Geometry check sheet. Reference: the model listing, model coordinates, mm. Face numbers are marked on the shaded views. A direction names the side the tool comes from. Coordinates: 2 decimals unless noted, no trailing zeros. Order: outer loops, then holes, each group sorted by start corner. A loop starts at its lowest first (then second) coordinate and runs counter-clockwise, first axis right, second up. Notation, with made-up numbers: (38.25, 68) - (96.25, 68) arc R13 cw to (96.25, 86) - close; hole circle Ø3 at (14.5, 17.25). An arc over 180 degrees is marked (long way). Use CSV: the item, a comma, the result in double quotes. Start each with the question number.
1) Sectioned sample at C-C, the plane z = 4. Record the cut outline in (x, y).
2) Thickness scan on probe 1 along X at (y, z) = (0.8, 19.5); probe 2 along Z at (x, y) = (-20, 1.9); probe 3 along Y at (x, z) = (17.5, -19.5). Record the ranges inside material, lowest first. Write a range as [from, to].
3) Sectioned sample at A-A, the plane y = 3.05. Record the cut outline in (x, z), and give its area (3 significant figures).
4) Depth check by flat-ended pin: P1, Ø0.6, axis at y = 2.5, z = -0.5, coming from the +X side; P2, Ø2.5, axis at x = 19.5, z = -19.5, coming from the +Y side. Enter the tip coordinate at first touch or a pass-through.
5) Tool access check on the marked faces 1 and 2. Record the directions out of +Z, -Z, +X, -X, +Y, -Y that give a thin tool (end or side, any length) a straight path to the whole face; none if there is none.
6) Sectioned sample at B-B, the plane y = 0.7. Record the cut outline in (x, z).
7) Sectioned sample at D-D, the plane x = 5.5. Record the cut outline in (y, z), and give its area (3 significant figures).
from build123d import *

# Parameters (mm, degrees)
SKETCH2_R           = 1.5
BOSS_EXTRUDE1_DEPTH = 2
BOSS_EXTRUDE2_DEPTH = 2
CUT_EXTRUDE1_DEPTH  = 2


with BuildPart() as part:
    # Sketch2 → Boss-Extrude1 (new body)
    with BuildSketch(Plane(origin=(0, 0, 0), x_dir=(1, 0, 0), z_dir=(0, 1, 0))):
        with BuildLine():
            Line((-19.5, 22.5), (19.5, 22.5))
            ThreePointArc((19.5, 22.5), (21.621320344, 21.621320344), (22.5, 19.5))
            Line((22.5, 19.5), (22.5, -19.5))
            ThreePointArc((22.5, -19.5), (21.621320344, -21.621320344), (19.5, -22.5))
            Line((19.5, -22.5), (-19.5, -22.5))
            ThreePointArc((-19.5, -22.5), (-21.621320344, -21.621320344), (-22.5, -19.5))
            Line((-22.5, -19.5), (-22.5, 19.5))
            ThreePointArc((-22.5, 19.5), (-21.621320344, 21.621320344), (-19.5, 22.5))
        make_face()
        with Locations(Location((19.5, -19.5, 0), (0, 0, 270))):
            Circle(SKETCH2_R, mode=Mode.SUBTRACT)
        with Locations(Location((19.5, 19.5, 0), (0, 0, 270))):
            Circle(SKETCH2_R, mode=Mode.SUBTRACT)
        with Locations(Location((-19.5, 19.5, 0), (0, 0, 270))):
            Circle(SKETCH2_R, mode=Mode.SUBTRACT)
        with Locations(Location((-19.5, -19.5, 0), (0, 0, 270))):
            Circle(SKETCH2_R, mode=Mode.SUBTRACT)
    extrude(amount=BOSS_EXTRUDE1_DEPTH)

    # Sketch3 → Boss-Extrude2 (add)
    with BuildSketch(Plane(origin=(0, 2, 0), x_dir=(1, 0, 0), z_dir=(0, 1, 0))):
        with BuildLine():
            Line((-11.653247837, 14.653247837), (11.653247837, 14.653247837))
            ThreePointArc((11.653247837, 14.653247837), (13.774568181, 13.774568181), (14.653247837, 11.653247837))
            Line((14.653247837, 11.653247837), (14.653247837, -11.653247837))
            ThreePointArc((14.653247837, -11.653247837), (13.774568181, -13.774568181), (11.653247837, -14.653247837))
            Line((11.653247837, -14.653247837), (-11.653247837, -14.653247837))
            ThreePointArc((-11.653247837, -14.653247837), (-13.774568181, -13.774568181), (-14.653247837, -11.653247837))
            Line((-14.653247837, -11.653247837), (-14.653247837, 11.653247837))
            ThreePointArc((-14.653247837, 11.653247837), (-13.774568181, 13.774568181), (-11.653247837, 14.653247837))
        make_face()
    extrude(amount=BOSS_EXTRUDE2_DEPTH)

    # Sketch4 → Cut-Extrude1 (cut)
    with BuildSketch(Plane(origin=(0, 4, 0), x_dir=(1, 0, 0), z_dir=(0, 1, 0))):
        with BuildLine():
            Line((11.675246151, -1.309846963), (1.675246151, -2.488684458))
            ThreePointArc((1.675246151, -2.488684458), (0, -3), (-1.675246151, -2.488684458))
            Line((-1.675246151, -2.488684458), (-11.675246151, -1.309846963))
            ThreePointArc((-11.675246151, -1.309846963), (-12.444287238, 0), (-11.675246151, 1.309846963))
            Line((-11.675246151, 1.309846963), (-1.675246151, 2.488684458))
            ThreePointArc((-1.675246151, 2.488684458), (0, 3), (1.675246151, 2.488684458))
            Line((1.675246151, 2.488684458), (11.675246151, 1.309846963))
            ThreePointArc((11.675246151, 1.309846963), (12.444287238, 0), (11.675246151, -1.309846963))
        make_face()
    extrude(amount=-CUT_EXTRUDE1_DEPTH, mode=Mode.SUBTRACT)


solid = part.part
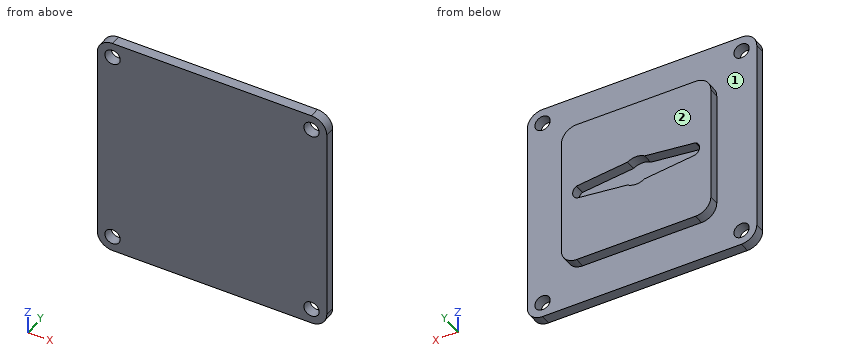
Evaluation:
1,outline,"(-22.5, 0) - (22.5, 0) - (22.5, 2) - (14.65, 2) - (14.65, 4) - (-14.65, 4) - (-14.65, 2) - (-22.5, 2) - close"
2,probe 1,"[-22.5, -21], [-18, 18], [21, 22.5]"
2,probe 2,"[-22.46, -20.91], [-18.09, 18.09], [20.91, 22.46]"
2,probe 3,"[0, 2]"
3,outline,"(-14.65, -11.65) arc R3 ccw to (-11.65, -14.65) - (11.65, -14.65) arc R3 ccw to (14.65, -11.65) - (14.65, 11.65) arc R3 ccw to (11.65, 14.65) - (-11.65, 14.65) arc R3 ccw to (-14.65, 11.65) - close; hole (-11.68, -1.31) - (-1.68, -2.49) arc R3 ccw to (1.68, -2.49) - (11.68, -1.31) arc R1.5 ccw to (11.68, 1.31) - (1.68, 2.49) arc R3 ccw to (-1.68, 2.49) - (-11.68, 1.31) arc R1.5 ccw to start"
3,area,"753 mm²"
4,P1,"x = 14.65"
4,P2,"through"
5,face 1,"+Y"
5,face 2,"+Z, -Z, +X, -X, +Y"
6,outline,"(-22.5, -19.5) arc R3 ccw to (-19.5, -22.5) - (19.5, -22.5) arc R3 ccw to (22.5, -19.5) - (22.5, 19.5) arc R3 ccw to (19.5, 22.5) - (-19.5, 22.5) arc R3 ccw to (-22.5, 19.5) - close; hole circle Ø3 at (-19.5, -19.5); hole circle Ø3 at (-19.5, 19.5); hole circle Ø3 at (19.5, -19.5); hole circle Ø3 at (19.5, 19.5)"
7,outline,"(0, -22.5) - (2, -22.5) - (2, -14.65) - (4, -14.65) - (4, -2.04) - (2, -2.04) - (2, 2.04) - (4, 2.04) - (4, 14.65) - (2, 14.65) - (2, 22.5) - (0, 22.5) - close"
7,area,"140 mm²"
